```python
from build123d import *

# Parameters (mm, degrees)
F0_R     = 3.25
F3_DEPTH = 18
F2_W     = 100
F2_H     = 80
F4_DEPTH = 15.5
F5_DEPTH = 25
F6_R     = 8


with BuildPart() as f3:
    # F0 (on Top) → F3 (new body)
    with BuildSketch(Plane.XY):
        with BuildLine():
            Line((-50, 42.5), (-50, -42.5))
            Line((-50, -42.5), (-40, -42.5))
            Line((-40, -42.5), (-40, -52.5))
            ThreePointArc((-40, -52.5), (-35, -57.5), (-30, -52.5))
            Line((-30, -52.5), (-30, -42.5))
            Line((-30, -42.5), (32.5, -42.5))
            Line((32.5, -42.5), (32.5, -52.5))
            ThreePointArc((32.5, -52.5), (37.5, -57.5), (42.5, -52.5))
            Line((42.5, -52.5), (42.5, -42.5))
            Line((42.5, -42.5), (52.5, -42.5))
            Line((52.5, -42.5), (52.5, 42.5))
            Line((52.5, 42.5), (42.5, 42.5))
            Line((42.5, 42.5), (42.5, 52.5))
            ThreePointArc((42.5, 52.5), (37.5, 57.5), (32.5, 52.5))
            Line((32.5, 52.5), (32.5, 42.5))
            Line((32.5, 42.5), (-30, 42.5))
            Line((-30, 42.5), (-30, 52.5))
            ThreePointArc((-30, 52.5), (-35, 57.5), (-40, 52.5))
            Line((-40, 52.5), (-40, 42.5))
            Line((-40, 42.5), (-50, 42.5))
        make_face()
        with Locations((-35, -52.5)):
            Circle(F0_R, mode=Mode.SUBTRACT)
        with Locations((37.5, -52.5)):
            Circle(F0_R, mode=Mode.SUBTRACT)
        with Locations((-35, 52.5)):
            Circle(F0_R, mode=Mode.SUBTRACT)
        with Locations((37.5, 52.5)):
            Circle(F0_R, mode=Mode.SUBTRACT)
    extrude(amount=-F3_DEPTH)

    # F2 (on face) → F4 (cut)
    with BuildSketch(Plane.XY):
        Rectangle(F2_W, F2_H)
    extrude(amount=-F4_DEPTH, mode=Mode.SUBTRACT)

    # F1 (on Top) → F5 (cut)
    with BuildSketch(Plane.XY):
        with BuildLine():
            Line((25, 25), (-25, 25))
            ThreePointArc((-25, 25), (-32.071068, 22.071068), (-35, 15))
            Line((-35, 15), (-35, -15))
            ThreePointArc((-35, -15), (-32.071068, -22.071068), (-25, -25))
            Line((-25, -25), (25, -25))
            ThreePointArc((25, -25), (32.071068, -22.071068), (35, -15))
            Line((35, -15), (35, 15))
            ThreePointArc((35, 15), (32.071068, 22.071068), (25, 25))
        make_face()
    extrude(amount=-F5_DEPTH, mode=Mode.SUBTRACT)

    # F6
    f6_edges = [f3.edges().sort_by_distance(p)[0] for p in [
        (-40, 42.5, -9),
        (32.5, 42.5, -9),
        (-40, -42.5, -9),
        (32.5, -42.5, -9),
        (42.5, -42.5, -9),
        (-30, -42.5, -9),
        (42.5, 42.5, -9),
        (-30, 42.5, -9),
    ]]
    fillet(f6_edges, radius=F6_R)


solid = f3.part
```
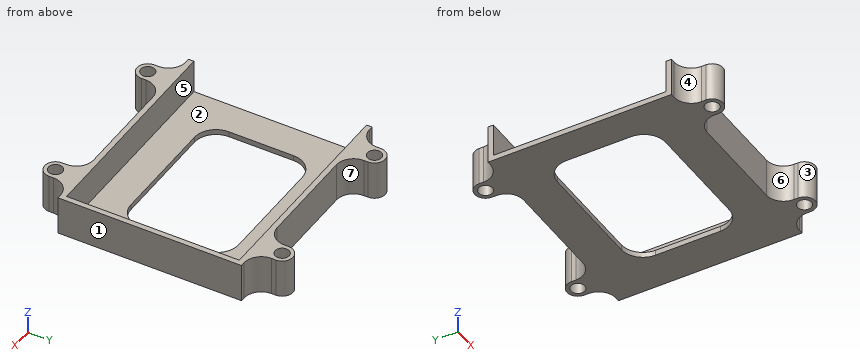
The model under review builds one solid part; all positions refer to its coordinate system, in mm. Face numbers are marked on the shaded views. A direction names the side the tool comes from. Round coordinates to 2 decimals unless told otherwise and drop trailing zeros. Order: outer loops, then holes, each group sorted by start corner. A loop starts at its lowest first (then second) coordinate and runs counter-clockwise, first axis right, second up. Notation, with made-up numbers: M 14,-17.75 L 57,-17.75 A12 ccw 57,-4.75 Z; hole C -35.75,20.5 d2. An arc over 180 degrees is marked long. Use a Markdown table: item, result.
1) Consider section B-B (y = -5). Write out the cut boundary in (x, z).
Report:
| item | result |
|---|---|
| outline | M -50,-18 L -35,-18 L -35,-15.5 L -50,-15.5 Z; M 35,-18 L 52.5,-18 L 52.5,0 L 50,0 L 50,-15.5 L 35,-15.5 Z |
2) Consider section A-A (x = 37.5). Write out the cut boundary in (y, z), then the cut area to 3 significant figures.
Report:
| item | result |
|---|---|
| outline | M -57.5,-18 L -55.75,-18 L -55.75,0 L -57.5,0 Z; M -49.25,-18 L 49.25,-18 L 49.25,0 L 40,0 L 40,-15.5 L -40,-15.5 L -40,0 L -49.25,0 Z; M 55.75,-18 L 57.5,-18 L 57.5,0 L 55.75,0 Z |
| area | 596 mm^2 |
3) Insertion check: pin 1 (2 mm diameter, centred on y = -51, z = -13, fed in from -X); pin 2 (1.5 mm diameter, centred on x = 5, z = -11, fed in from +Y); pin 3 (5 mm diameter, centred on x = -19.5, z = -3.5, fed in from -Y); pin 4 (1.5 mm diameter, centred on x = 0, y = -42, fed in from +Z). Each pin has a flat end and moves straight along its axis. Give the tip position at first contact, or say it passes through.
Report:
| item | result |
|---|---|
| pin 1 | x = -40.02 |
| pin 2 | y = 42.5 |
| pin 3 | y = -42.5 |
| pin 4 | z = 0 |
4) Wall thickness on line 1 along Y through (x, z) = (37.5, -9); line 2 along Y through (x, z) = (-10, -13.25); line 3 along Z through (x, y) = (-42, -12): over which ranges is each line inside the solid? List them lowest first. Write a range as [from, to].
Report:
| item | result |
|---|---|
| line 1 | [-57.5, -55.75], [-49.25, -40], [40, 49.25], [55.75, 57.5] |
| line 2 | [-42.5, -40], [40, 42.5] |
| line 3 | [-18, -15.5] |
5) Consider section D-D (y = 18.5). Write out the cut boundary in (x, z).
Report:
| item | result |
|---|---|
| outline | M -50,-18 L -34.37,-18 L -34.37,-15.5 L -50,-15.5 Z; M 34.37,-18 L 52.5,-18 L 52.5,0 L 50,0 L 50,-15.5 L 34.37,-15.5 Z |
6) Draft analysis for pull direction X (two halves, no side actions). For the marked faces 1, 2, 3 and 4, state which applies: released by +X, released by -X, zero draft, split by the parting line, or undercut.
Report:
| item | result |
|---|---|
| face 1 | released by +X |
| face 2 | zero draft |
| face 3 | undercut |
| face 4 | released by -X |
7) Tool access review of the marked faces 5, 6 and 7: name each direction out of +Z, -Z, +X, -X, +Y, -Y from which nothing blocks a thin tool from reaching the whole face with its end or side.
Report:
| item | result |
|---|---|
| face 5 | +Z, -X |
| face 6 | +Z, -Z, -Y |
| face 7 | +Z, -Z, +Y |
8) Consider section C-C (y = -27.5). Write out the cut boundary in (x, z), then the cut area to 3 significant figures.
Report:
| item | result |
|---|---|
| outline | M -50,-18 L 52.5,-18 L 52.5,0 L 50,0 L 50,-15.5 L -50,-15.5 Z |
| area | 295 mm^2 |
